The model under review builds one solid part; all positions refer to its coordinate system, in mm. A direction names the side the tool comes from. Round coordinates to 2 decimals unless told otherwise and drop trailing zeros. Loops run counter-clockwise (first coordinate to the right, second up) from the corner with the lowest first, then second, coordinate; pieces in that order, holes last. Notation, with made-up numbers: M 79.25,53.25 L 119.25,53.25 A23 ccw 119.25,67.25 Z; hole C -4,38.5 d7. An arc over 180 degrees is marked long. Answer in a Markdown table with one row per item. Add a question column.
from build123d import *
from build123d import SkipClean  # not in build123d's __all__

# Parameters (mm, degrees)
F0_R      = 20.15
F0_R_2    = 14.15
F1_DEPTH  = 350
F2_R      = 5.75
F3_DEPTH  = 25
F5_DEPTH  = 195
F6_DEPTH  = 350.0010001
F7_R      = 5.75
F8_DEPTH  = 20.15
F9_R      = 8.5
F10_DEPTH = 2
F11_DEPTH = 25


with BuildPart() as f1:
    # F0 (on Top) → F1 (new body)
    with BuildSketch(Plane.XY):
        Circle(F0_R)
        Circle(F0_R_2, mode=Mode.SUBTRACT)
    extrude(amount=F1_DEPTH)

    # F2 (on Front) → F3 (cut)
    with BuildSketch(Plane.XZ):
        with Locations((0, 320)):
            Circle(F2_R)
        with Locations((0, 270)):
            Circle(F2_R)
        with Locations((0, 220)):
            Circle(F2_R)
        with Locations((0, 170)):
            Circle(F2_R)
    extrude(amount=F3_DEPTH, mode=Mode.SUBTRACT)

    # F4 (on face) → F5 (cut)
    with BuildSketch(Plane.XY.offset(350)):
        with BuildLine():
            Line((-7.5, -21.5977942477), (7.5, -21.5977942477))
            Line((7.5, -21.5977942477), (7.5, -18.7022057523))
            ThreePointArc((7.5, -18.7022057523), (0, -20.15), (-7.5, -18.7022057523))
            Line((-7.5, -18.7022057523), (-7.5, -21.5977942477))
        make_face()
        with BuildLine():
            ThreePointArc((-7.5, -18.7022057523), (0, -20.15), (7.5, -18.7022057523))
            Line((7.5, -18.7022057523), (-7.5, -18.7022057523))
        make_face()
    extrude(amount=-F5_DEPTH, mode=Mode.SUBTRACT)

    # F4 (on face) → F6 (cut, through all)
    with BuildSketch(Plane.XY.offset(350)):
        with BuildLine():
            ThreePointArc((5.7980718495, 19.2977942477), (0, 20.15), (-5.7980718495, 19.2977942477))
            Line((-5.7980718495, 19.2977942477), (5.7980718495, 19.2977942477))
        make_face()
    extrude(amount=-F6_DEPTH, mode=Mode.SUBTRACT)

    # F7 (on Right) → F8 (join)
    with BuildSketch(Plane.YZ):
        with Locations((0, 15)):
            Circle(F7_R)
        with Locations((0, 155)):
            Circle(F7_R)
    with SkipClean():  # cleaning this boolean's faces spoils the solid; the shape is the same uncleaned
        extrude(amount=F8_DEPTH)

    # F9 (on face) → F10 (cut)
    with BuildSketch(Plane.YZ.offset(20.15)):
        with Locations((0, 155)):
            Circle(F9_R)
        with BuildLine():
            ThreePointArc((5.75, 155), (4.0658639918, 150.9341360082), (0, 149.25))
            ThreePointArc((0, 149.25), (-5.75, 155), (0, 160.75))
            ThreePointArc((0, 160.75), (4.0658639918, 159.0658639918), (5.75, 155))
        make_face(mode=Mode.SUBTRACT)
        with BuildLine():
            ThreePointArc((0, 160.75), (-5.75, 155), (0, 149.25))
            Line((0, 149.25), (0, 160.75))
        make_face()
        with Locations((0, 15)):
            Circle(F9_R)
    with SkipClean():  # cleaning this boolean's faces spoils the solid; the shape is the same uncleaned
        extrude(amount=-F10_DEPTH, mode=Mode.SUBTRACT)

    # F7 (on Right) → F11 (cut)
    with BuildSketch(Plane.YZ):
        with Locations((0, 15)):
            Circle(F7_R)
        with Locations((0, 155)):
            Circle(F7_R)
    extrude(amount=F11_DEPTH, mode=Mode.SUBTRACT)


solid = f1.part
1. Take a section at C-C, the plane z = 70. State the section outline as (x, y) points, and give its area (3 significant figures).
2. Take a section at A-A, the plane x = 0. State the section outline as (y, z) points, and give its area (3 significant figures).
3. Take a section at B-B, the plane z = 170. State the section outline as (x, y) points, and give its area (3 significant figures).
4. Take a section at D-D, the plane z = 15. State the section outline as (x, y) points.
5. Mouldability with a two-part tool opening along X and no side actions: class faces 6 (the cylindrical face through (-10.43, 9.56, 172.55)), 7 (the flat face through (18.15, 2, 9)), 8 (the cylindrical face through (3.09, -15.78, 274.85)), 9 (the flat face through (0, 19.298, 177)) as released by +X, released by -X, zero draft, split by the parting line, or undercut.
6. To check wall thickness, follow probe 1 along Z at (x, y) = (0, -17); probe 2 along Z at (x, y) = (19.1, 0); probe 3 along Y at (x, z) = (0, 319.5). State the ranges of each line that lie inside material, in increasing order.
7. For pin 1 Ø15 at (y, z) = (0, 155) entering from +X; pin 2 Ø8.5 at (y, z) = (4, 157) entering from +X; pin 3 Ø6 at (x, z) = (-10, 303.5) entering from +Y; pin 4 Ø17 at (x, y) = (0, 0) entering from +Z, all flat-tipped, find the tip position at first contact; note any pin that passes through.
8. Machinability: for faces 1 (the cylindrical face through (3.09, -15.78, 174.85)), 2 (the cylindrical face through (-12.563, -15.754, 172.55)), 3 (the flat face through (0, -18.702, 254)), 4 (the cylindrical face through (16.083, 5.312, 152.798)), 5 (the flat face through (-14, -4, 350)), which of the approach directions +Z, -Z, +X, -X, +Y, -Y give a long, thin tool a straight path to every point of the face, cutting with its end or side? Answer none if there is none.
Check sheet entries:
| question | item | result |
|---|---|---|
| 1 | outline | M -5.8,19.3 A20.15 ccw long 5.8,19.3 Z; hole C 0,0 d28.3 |
| 1 | area | 640 mm^2 |
| 2 | outline | M -20.15,0 L -14.15,0 L -14.15,164.25 L -18.7,164.25 L -18.7,155 L -20.15,155 Z; M -18.7,175.75 L -14.15,175.75 L -14.15,214.25 L -18.7,214.25 Z; M -18.7,225.75 L -14.15,225.75 L -14.15,264.25 L -18.7,264.25 Z; M -18.7,275.75 L -14.15,275.75 L -14.15,314.25 L -18.7,314.25 Z; M -18.7,325.75 L -14.15,325.75 L -14.15,350 L -18.7,350 Z; M 14.15,0 L 19.3,0 L 19.3,350 L 14.15,350 Z |
| 2 | area | 3,410 mm^2 |
| 3 | outline | M -7.5,-18.7 L -5.75,-18.7 L -5.75,-12.93 A14.15 cw long 5.75,-12.93 L 5.75,-18.7 L 7.5,-18.7 A20.15 ccw 5.8,19.3 L -5.8,19.3 A20.15 ccw Z |
| 3 | area | 568 mm^2 |
| 4 | outline | M -5.8,19.3 A20.15 ccw long 18.27,-8.5 L 18.15,-8.5 L 18.15,-5.75 L 12.93,-5.75 A14.15 cw long 12.93,5.75 L 18.15,5.75 L 18.15,8.5 L 18.27,8.5 A20.15 ccw 5.8,19.3 Z |
| 5 | face 6 | undercut |
| 5 | face 7 | released by +X |
| 5 | face 8 | undercut |
| 5 | face 9 | zero draft |
| 6 | probe 1 | z = 0 to 164.25, 175.75 to 214.25, 225.75 to 264.25, 275.75 to 314.25, 325.75 to 350 |
| 6 | probe 2 | z = 0 to 6.5, 23.5 to 146.5, 163.5 to 350 |
| 6 | probe 3 | y = 14.15 to 19.3 |
| 7 | pin 1 | stops at x = 18.15 |
| 7 | pin 2 | stops at x = 19.04 |
| 7 | pin 3 | stops at y = 18.9 |
| 7 | pin 4 | passes through |
| 8 | face 1 | -Y |
| 8 | face 2 | +Z, -Z |
| 8 | face 3 | +Z, +X, -X, -Y |
| 8 | face 4 | +X |
| 8 | face 5 | +Z, +X, -X, +Y, -Y |
